Read the model definition and answer for the solid it produces. Units are mm, in the model's axes. Give positions to 0.01 mm unless a question says otherwise; leave off trailing zeros. Loops run counter-clockwise (first coordinate to the right, second up) from the corner with the lowest first, then second, coordinate; pieces in that order, holes last.
(1) Find section A-A, the plane z = -244. Write down the section's boundary in (x, y).
(2) Straight lines are drawn through the part: probe 1 along Y at (x, z) = (70.5, -400); probe 2 along Y at (x, z) = (28, -281); probe 3 along Z at (x, y) = (47, 35). For each, find the intervals that lie inside material, in ascending order.
(3) Each of these flat-tipped pins is pushed along its axis until it touches: P1, Ø8, axis at x = 127, y = 28, coming from the -Z side; P2, Ø5, axis at x = 98, z = -49.5, coming from the -Y side; P3, Ø12, axis at x = 40.5, z = -159.5, coming from the +Y side. Where does it stop, or does it pass through?
```python
from build123d import *

# Parameters (mm, degrees)
BOSS_EXTRUDE1_DEPTH = 455
FILLET1_R           = 10
FILLET2_R           = 10
FILLET3_R           = 10
FILLET4_R           = 10


with BuildPart() as part:
    # Sketch1 → Boss-Extrude1 (new body)
    with BuildSketch(Plane.XY):
        Polygon((0, 0), (155, 0), (155, 19), (0, 44), align=None)
    extrude(amount=-BOSS_EXTRUDE1_DEPTH)

    # Fillet1
    fillet1_edges = [part.edges().sort_by_distance(p)[0] for p in [
        (155, 19, -227.5),
    ]]
    fillet(fillet1_edges, radius=FILLET1_R)

    # Fillet2
    fillet2_edges = [part.edges().sort_by_distance(p)[0] for p in [
        (0, 44, -227.5),
    ]]
    fillet(fillet2_edges, radius=FILLET2_R)

    # Fillet3
    fillet3_edges = [part.edges().sort_by_distance(p)[0] for p in [
        (79.092324388, 31.243173486, 0),
        (152.613253046, 16.967366458, 0),
        (0, 16.128929526, 0),
        (3.516299046, 39.871112099, 0),
        (155, 5.241832752, 0),
    ]]
    fillet(fillet3_edges, radius=FILLET3_R)

    # Fillet4
    fillet4_edges = [part.edges().sort_by_distance(p)[0] for p in [
        (155, 5.241832752, -455),
        (79.092324388, 31.243173486, -455),
        (152.613253046, 16.967366458, -455),
        (0, 16.128929526, -455),
        (3.516299046, 39.871112099, -455),
    ]]
    fillet(fillet4_edges, radius=FILLET4_R)


solid = part.part
```
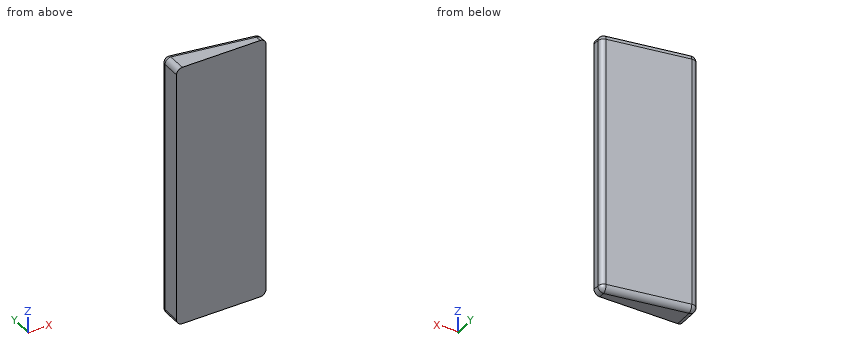
Entries:
1. outline: (0, 0) - (155, 0) - (155, 10.48) arc R10 ccw to (146.59, 20.36) - (11.59, 42.13) arc R10 ccw to (0, 32.26) - close
2. probe 1: y = 0 to 32.63
2. probe 2: y = 0 to 39.48
2. probe 3: z = -450.11 to -4.89
3. P1: passes through
3. P2: stops at y = 0
3. P3: stops at y = 38.44
